Build history of the part. All positions in model axes, mm. A direction names the side the tool comes from. Give positions to 0.01 mm unless a question says otherwise; leave off trailing zeros. Order: outer loops, then holes, each group sorted by start corner. A loop starts at its lowest first (then second) coordinate and runs counter-clockwise, first axis right, second up. Notation, with made-up numbers: M -11,-7.5 L 35,-7.5 A27 cw 35,15.5 Z; hole C 51,68 d7. An arc over 180 degrees is marked long. One line per item, written item: value.
from build123d import *

# Parameters (mm, degrees)
BOSS_EXTRUDE1_DEPTH = 19.05
CUT_EXTRUDE1_DEPTH  = 20.05
SKETCH2_4_W         = 12.954
SKETCH2_4_H         = 1.7018
CUT_EXTRUDE2_DEPTH  = 18.25625
SKETCH6_W           = 0.608326788
SKETCH6_H           = 1.5875
SKETCH8_W           = 2.576826788
SKETCH8_H           = 1.5875
SKETCH9_W           = 12.954
SKETCH9_H           = 5.08
SKETCH9_H_2         = 2.159
CUT_EXTRUDE3_DEPTH  = 6.35


with BuildPart() as part:
    # Sketch1 → Boss-Extrude1 (new body)
    with BuildSketch(Plane(origin=(0, 0, 0), x_dir=(1, 0, 0), z_dir=(0, 1, 0))):
        with BuildLine():
            Line((-0.79375, 9.109483901), (-0.79375, 8.535673212))
            ThreePointArc((-0.79375, 8.535673212), (-7.424002774, 4.28625), (-7.78898484, -3.580428942))
            Line((-7.78898484, -3.580428942), (-8.285919473, -3.867334286))
            ThreePointArc((-8.285919473, -3.867334286), (-7.918936292, -4.572), (-7.492169473, -5.242149615))
            Line((-7.492169473, -5.242149615), (-6.99523484, -4.95524427))
            ThreePointArc((-6.99523484, -4.95524427), (0, -8.5725), (6.99523484, -4.95524427))
            Line((6.99523484, -4.95524427), (7.492169473, -5.242149615))
            ThreePointArc((7.492169473, -5.242149615), (7.918936292, -4.572), (8.285919473, -3.867334286))
            Line((8.285919473, -3.867334286), (7.78898484, -3.580428942))
            ThreePointArc((7.78898484, -3.580428942), (7.424002774, 4.28625), (0.79375, 8.535673212))
            Line((0.79375, 8.535673212), (0.79375, 9.109483901))
            ThreePointArc((0.79375, 9.109483901), (0, 9.144), (-0.79375, 9.109483901))
        make_face()
    extrude(amount=BOSS_EXTRUDE1_DEPTH)

    # Sketch2 → Cut-Extrude1 (cut, through all)
    with BuildSketch(Plane(origin=(0, 19.05, 0), x_dir=(1, 0, 0), z_dir=(0, 1, 0))):
        with BuildLine():
            Line((-4.543615348, 4.303093955), (-3.175, 2.4638))
            Line((-3.175, 2.4638), (3.175, 2.4638))
            Line((3.175, 2.4638), (4.543615348, 4.303093955))
            ThreePointArc((4.543615348, 4.303093955), (4.598203733, 4.928342625), (4.064, 5.2578))
            Line((4.064, 5.2578), (-4.064, 5.2578))
            ThreePointArc((-4.064, 5.2578), (-4.598203733, 4.928342625), (-4.543615348, 4.303093955))
        make_face()
    extrude(amount=-CUT_EXTRUDE1_DEPTH, mode=Mode.SUBTRACT)

    # Sketch2_4 → Cut-Extrude2 (cut)
    with BuildSketch(Plane(origin=(0, 19.05, 0), x_dir=(1, 0, 0), z_dir=(0, 1, 0))):
        with Locations((0, 1.6129)):
            Rectangle(SKETCH2_4_W, SKETCH2_4_H)
    extrude(amount=-CUT_EXTRUDE2_DEPTH, mode=Mode.SUBTRACT)

    # Sketch6 → Cut-Revolve2 (revolve, cut)
    with BuildSketch(Plane(origin=(0, 0, 0), x_dir=(0, 0, -1), z_dir=(1, 0, 0))):
        with Locations((8.839836606, 0.79375)):
            Rectangle(SKETCH6_W, SKETCH6_H)
    revolve(axis=Axis((0, 19.730213777, 0), (0, -1, 0)), mode=Mode.SUBTRACT)

    # Sketch8 → Revolve2 (revolve)
    with BuildSketch(Plane(origin=(0, 0, 0), x_dir=(0, 0, -1), z_dir=(1, 0, 0))):
        with Locations((9.824086606, 0.79375)):
            Rectangle(SKETCH8_W, SKETCH8_H)
    revolve(axis=Axis((0, 4.48386458, 0), (0, -1, 0)))

    # Sketch9 → Cut-Extrude3 (cut)
    with BuildSketch(Plane(origin=(0, 19.05, 0), x_dir=(1, 0, 0), z_dir=(0, 1, 0))):
        with Locations((0, -1.778)):
            Rectangle(SKETCH9_W, SKETCH9_H)
        with Locations((0, 3.5433)):
            Rectangle(SKETCH9_W, SKETCH9_H_2)
    extrude(amount=-CUT_EXTRUDE3_DEPTH, mode=Mode.SUBTRACT)


solid = part.part
1) Saw through at D-D, the plane z = 0. Write the cut outline in (x, y).
Check values:
outline: M -11.11,0 L 11.11,0 L 11.11,1.59 L 8.57,1.59 L 8.57,19.05 L 6.48,19.05 L 6.48,12.7 L -6.48,12.7 L -6.48,19.05 L -8.57,19.05 L -8.57,1.59 L -11.11,1.59 Z
2) Pin check, flat tips, straight feed: pin 1 (9.5 mm diameter, centred on x = -3, y = 7.5, fed in from -Z); pin 2 (0.6 mm diameter, centred on y = 9.5, z = -9, fed in from -X); pin 3 (2.5 mm diameter, centred on y = 5.5, z = -0.5, fed in from +X). Stop position of each tip, or through.
Check values:
pin 1: z = -9.14
pin 2: x = -0.79
pin 3: x = 8.57
3) Tool access for faces 1 (the face through (-7.924, 10.197, 4.562)), 2 (the face through (-3.87, 6.44, -3.4)), 3 (the face through (-0.11, 10.2, 8.57)), 4 (the face through (0, 16, 4.318)), 5 (the face through (-7.366, 10.197, -4.385)): list every direction of +Z, -Z, +X, -X, +Y, -Y with a clear straight run to the whole face (end or side of a thin tool).
Check values:
face 1: +Z, -X, +Y
face 2: +Y, -Y
face 3: +Z, +Y
face 4: +Y
face 5: -X, +Y
4) Saw through at C-C, the plane z = -3.25. Write the cut outline in (x, y).
Check values:
outline: M -10.63,0 L -3.76,0 L -3.76,12.7 L -6.48,12.7 L -6.48,19.05 L -7.93,19.05 L -7.93,1.59 L -10.63,1.59 Z; M 3.76,0 L 10.63,0 L 10.63,1.59 L 7.93,1.59 L 7.93,19.05 L 6.48,19.05 L 6.48,12.7 L 3.76,12.7 Z
5) Drill centre lines: probe 1 along Y at (x, z) = (-9.75, -4.75); probe 2 along X at (y, z) = (14.75, -0.25); probe 3 along Z at (x, y) = (4.25, 5.75). Where is each one in solid material? Low to high. Write a range as from..to.
Check values:
probe 1: 0..1.59
probe 2: -8.57..-6.48, 6.48..8.57
probe 3: -7.44..-5.23, -3.91..-2.46, -0.76..7.44
6) Saw through at B-B, the plane y = 14.5. Write the cut outline in (x, z) (1 decimal).
Check values:
outline: M -8.3,3.9 L -7.8,3.6 A8.6 ccw -0.8,-8.5 L -0.8,-9.1 A9.1 ccw 0.8,-9.1 L 0.8,-8.5 A8.6 ccw 7.8,3.6 L 8.3,3.9 A9.1 ccw 7.5,5.2 L 7,5 A8.6 ccw -7,5 L -7.5,5.2 A9.1 ccw Z; hole M -6.5,-4.6 L -4.7,-4.6 A0.6 ccw -4.1,-5.3 L 4.1,-5.3 A0.6 ccw 4.7,-4.6 L 6.5,-4.6 L 6.5,4.3 L -6.5,4.3 Z
7) Saw through at A-A, the plane x = 0. Write the cut outline in (y, z), then the cut area to 3 significant figures.
Check values:
outline: M 0,-11.11 L 1.59,-11.11 L 1.59,-9.14 L 19.05,-9.14 L 19.05,-5.26 L 0,-5.26 Z; M 0,-2.46 L 0.79,-2.46 L 0.79,-0.76 L 12.7,-0.76 L 12.7,4.32 L 19.05,4.32 L 19.05,8.57 L 1.59,8.57 L 1.59,11.11 L 0,11.11 Z
area: 228 mm^2
8) Mould opens along X. For faces 6 (the face through (5, 7, -2.464)), 7 (the face through (3.34, 0.8, -10.6)), 8 (the face through (1, 19.05, 5)), 9 (the face through (-4.59, 9.66, -4.94)) say: released by +X, released by -X, zero draft, split by the parting line, or undercut.
Check values:
face 6: undercut
face 7: split by the parting line
face 8: zero draft
face 9: undercut
